```python
from build123d import *

# Parameters (mm, degrees)
REJFNING_0_5_X_45_GR_SIZE = 0.5
RUNDING_R1_R              = 1
HOLE1_D                   = 8.5
HOLE1_DEPTH               = 17.5
HOLE1_TIP                 = 2.553657631


with BuildPart() as part:
    # Sketch1 → Base-Revolve (revolve)
    with BuildSketch(Plane.XY):
        Polygon((0, 9.5), (35, 9.5), (35, 15), (37, 15), (37, 20), (32, 20), (32, 40), (7.309401077, 40), (5, 36), (2, 36), (2, 35), (0, 35), align=None)
    revolve(axis=Axis((-31.276903974, 0, 0), (1, 0, 0)))

    # Rejfning 0,5 x 45 gr.
    rejfning_0_5_x_45_gr_edges = [part.edges().sort_by_distance(p)[0] for p in [
        (37, -20, 0),
    ]]
    chamfer(rejfning_0_5_x_45_gr_edges, length=REJFNING_0_5_X_45_GR_SIZE)

    # Runding R1
    runding_r1_edges = [part.edges().sort_by_distance(p)[0] for p in [
        (32, -40, 0),
    ]]
    fillet(runding_r1_edges, radius=RUNDING_R1_R)

    # Hole1
    with Locations(Plane(origin=(32, 0, 0), x_dir=(0, 0, -1), z_dir=(1, 0, 0))):
        with Locations((0, 28), (-28, 0), (0, -28), (28, 0)):
            Hole(HOLE1_D / 2, depth=HOLE1_DEPTH)
            with Locations((0, 0, -(HOLE1_DEPTH + HOLE1_TIP / 2))):  # 118° drill point
                Cone(0, HOLE1_D / 2, HOLE1_TIP, mode=Mode.SUBTRACT)


solid = part.part
```
Here's how the part is built. I have some questions about the finished solid (model axes, mm). A direction names the side the tool comes from. Round coordinates to 2 decimals unless told otherwise and drop trailing zeros. Order: outer loops, then holes, each group sorted by start corner. A loop starts at its lowest first (then second) coordinate and runs counter-clockwise, first axis right, second up. Notation, with made-up numbers: (62.25, 45) -> (102.25, 45) arc R27 cw to (102.25, 64) -> close; hole circle Ø2 at (-23.5, -30). An arc over 180 degrees is marked (long way). Use a Markdown table: item, result. Add a question column.
(1) For faces 4 (the face through (3.479, -4.686, 35.694)), 5 (the face through (23.127, 0.187, 23.754)), 6 (the face through (0, 7, -7)), which set-ups out of +Z, -Z, +X, -X, +Y, -Y let a thin tool reach every point of the face, with its end or its side?
(2) Suppose I cut it at A-A, the plane x = 28.5. Please give me the cut outline in (y, z), and give its area (3 significant figures).
(3) I need wall thicknesses on line 1 along Z through (x, y) = (35.55, 0); line 2 along X through (y, z) = (32.5, 5); line 3 along Z through (x, y) = (19, 30). Which ranges of each line are inside material? Lowest first, please.
(4) For pin 1 Ø15 at (y, z) = (2.5, -0.5) entering from +X; pin 2 Ø10 at (y, z) = (-28, 0) entering from -X; pin 3 Ø5 at (x, z) = (9.5, -30) entering from +Y; pin 4 Ø12 at (x, z) = (17.5, 15) entering from -Y, each with a flat end and sliding along its axis, tell me the tip position at first contact or that it passes through.
(5) If we mould it in two halves opening along Y, with no side actions, what happens to faces 1 (the face through (23.13, -32.15, -0.92)), 2 (the face through (18.99, -8.67, -39.05)), 3 (the face through (37, -10, -11.5))? For each: released by +Y, released by -Y, zero draft, split by the parting line, or undercut.
(6) Suppose I cut it at B-B, the plane x = 10. Please give me the cut outline in (y, z), and give its area (3 significant figures).
Verdict:
| question | item | result |
|---|---|---|
| 1 | face 4 | -X |
| 1 | face 5 | +X |
| 1 | face 6 | +Z, -Z, -X, +Y, -Y |
| 2 | outline | circle Ø80 at (0, 0); hole circle Ø8.5 at (-28, 0); hole circle Ø19 at (0, 0); hole circle Ø8.5 at (0, -28); hole circle Ø8.5 at (0, 28); hole circle Ø8.5 at (28, 0) |
| 2 | area | 4,520 mm2 |
| 3 | line 1 | -20 to -15, 15 to 20 |
| 3 | line 2 | 0 to 32 |
| 3 | line 3 | -26.46 to -3.75, 3.75 to 26.46 |
| 4 | pin 1 | x = 35 |
| 4 | pin 2 | x = 0 |
| 4 | pin 3 | y = 29.05 |
| 4 | pin 4 | y = -38.97 |
| 5 | face 1 | undercut |
| 5 | face 2 | split by the parting line |
| 5 | face 3 | zero draft |
| 6 | outline | circle Ø80 at (0, 0); hole circle Ø19 at (0, 0) |
| 6 | area | 4,740 mm2 |
